Read the model definition and answer for the solid it produces. Units are mm, in the model's axes. Round coordinates to 2 decimals unless told otherwise and drop trailing zeros. Loops run counter-clockwise (first coordinate to the right, second up) from the corner with the lowest first, then second, coordinate; pieces in that order, holes last. Notation, with made-up numbers: (2, 20.25) - (23, 20.25) arc R37 ccw to (23, 56.25) - close; hole circle Ø3 at (-7, 54.5). An arc over 180 degrees is marked (long way). Use one line per item in the form item = value. Start each with the question number.
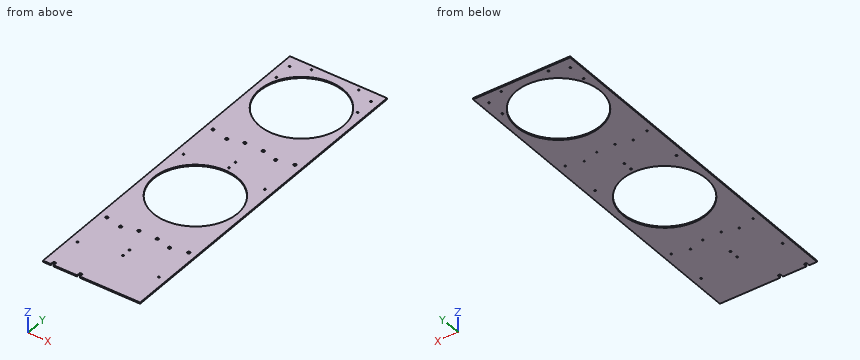
```python
from build123d import *

# Parameters (mm, degrees)
SKETCH1_W                                     = 469.9
SKETCH1_H                                     = 2413
SKETCH1_R                                     = 203.2
BOSS_EXTRUDE1_DEPTH                           = 6.35
CSK_FOR_1_4_FLAT_HEAD_SOCKET_CAP_SCR_2_COUNT  = 2
CSK_FOR_1_4_FLAT_HEAD_SOCKET_CAP_SCR_2_PITCH  = 76.2
CSK_FOR_1_4_FLAT_HEAD_SOCKET_CAP_SCR_3_COUNT  = 2
CSK_FOR_1_4_FLAT_HEAD_SOCKET_CAP_SCR_3_PITCH  = 89.142542345
CSK_FOR_1_4_FLAT_HEAD_SOCKET_CAP_SCR_4_COUNT  = 2
CSK_FOR_1_4_FLAT_HEAD_SOCKET_CAP_SCR_4_PITCH  = 163.936718394
CSK_FOR_1_4_FLAT_HEAD_SOCKET_CAP_SCR_5_COUNT  = 2
CSK_FOR_1_4_FLAT_HEAD_SOCKET_CAP_SCR_5_PITCH  = 711.2
CSK_FOR_1_4_FLAT_HEAD_SOCKET_CAP_SCR_6_COUNT  = 2
CSK_FOR_1_4_FLAT_HEAD_SOCKET_CAP_SCR_6_PITCH  = 695.384275934
CSK_FOR_1_4_FLAT_HEAD_SOCKET_CAP_SCR_7_COUNT  = 2
CSK_FOR_1_4_FLAT_HEAD_SOCKET_CAP_SCR_7_PITCH  = 716.764837904
CSK_FOR_1_4_FLAT_HEAD_SOCKET_CAP_SCR_8_COUNT  = 2
CSK_FOR_1_4_FLAT_HEAD_SOCKET_CAP_SCR_8_PITCH  = 710.371803251
CSK_FOR_1_4_FLAT_HEAD_SOCKET_CAP_SCR_9_COUNT  = 2
CSK_FOR_1_4_FLAT_HEAD_SOCKET_CAP_SCR_9_PITCH  = 1422.4
CSK_FOR_1_4_FLAT_HEAD_SOCKET_CAP_SCR_10_COUNT = 2
CSK_FOR_1_4_FLAT_HEAD_SOCKET_CAP_SCR_10_PITCH = 1404.60778242
CSK_FOR_1_4_FLAT_HEAD_SOCKET_CAP_SCR_11_COUNT = 2
CSK_FOR_1_4_FLAT_HEAD_SOCKET_CAP_SCR_11_PITCH = 1425.190567207
CSK_FOR_1_4_FLAT_HEAD_SOCKET_CAP_SCR_12_COUNT = 2
CSK_FOR_1_4_FLAT_HEAD_SOCKET_CAP_SCR_12_PITCH = 1412.087755797
CSK_FOR_1_4_FLAT_HEAD_SOCKET_CAP_SCR_13_COUNT = 2
CSK_FOR_1_4_FLAT_HEAD_SOCKET_CAP_SCR_13_PITCH = 153.55813077
CSK_FOR_1_4_FLAT_HEAD_SOCKET_CAP_SCR_14_COUNT = 2
CSK_FOR_1_4_FLAT_HEAD_SOCKET_CAP_SCR_14_PITCH = 242.697219812
CSK_FOR_1_4_FLAT_HEAD_SOCKET_CAP_SCR_15_COUNT = 2
CSK_FOR_1_4_FLAT_HEAD_SOCKET_CAP_SCR_15_PITCH = 749.86024568
CSK_FOR_1_4_FLAT_HEAD_SOCKET_CAP_SCR_16_COUNT = 2
CSK_FOR_1_4_FLAT_HEAD_SOCKET_CAP_SCR_16_PITCH = 1441.280581843
CSK_FOR_1_4_FLAT_HEAD_SOCKET_CAP_SCR_17_COUNT = 2
CSK_FOR_1_4_FLAT_HEAD_SOCKET_CAP_SCR_17_PITCH = 1428.974413563
CSK_FOR_1_4_FLAT_HEAD_SOCKET_CAP_SCR_18_COUNT = 2
CSK_FOR_1_4_FLAT_HEAD_SOCKET_CAP_SCR_18_PITCH = 725.925992834
F_5_16_0_3125_DIAMETER_HOLE1_D                = 7.9375
SKETCH6_W                                     = 469.9
SKETCH6_H                                     = 758.19
CUT_EXTRUDE1_DEPTH                            = 7.35
SKETCH8_W                                     = 13.208
SKETCH8_H                                     = 19.05
CUT_EXTRUDE2_DEPTH                            = 7.35
FILLET1_R                                     = 3.175


with BuildPart() as part:
    # Sketch1 → Boss-Extrude1 (new body)
    with BuildSketch(Plane.XY):
        with Locations((0, 1206.5)):
            Rectangle(SKETCH1_W, SKETCH1_H)
        with Locations((0, 695.96)):
            Circle(SKETCH1_R, mode=Mode.SUBTRACT)
        with Locations((0, 1407.16)):
            Circle(SKETCH1_R, mode=Mode.SUBTRACT)
        with Locations((0, 2118.36)):
            Circle(SKETCH1_R, mode=Mode.SUBTRACT)
    extrude(amount=BOSS_EXTRUDE1_DEPTH)

    # Sketch3 → CSK for 1/4 Flat Head Socket Cap Screw1 (revolve, cut)
    with BuildSketch(Plane(origin=(44.571271172, 378.545152647, 6.35), x_dir=(0, -1, 0), z_dir=(1, 0, 0))):
        Polygon((0, 0), (0, 6.35), (3.3782, 6.35), (3.3782, 3.871564875), (6.7437, 0), align=None)
    csk_for_1_4_flat_head_socket_cap_screw1 = revolve(axis=Axis((44.571271172, 378.545152647, 12.7), (0, 0, -1)), mode=Mode.SUBTRACT)

    # CSK for 1_4 Flat Head Socket Cap Scr 2: CSK for 1/4 Flat Head Socket Cap Screw1 ×2
    with Locations(*[Vector(0.965925826, -0.258819045, 0) * (i * CSK_FOR_1_4_FLAT_HEAD_SOCKET_CAP_SCR_2_PITCH) for i in range(1, CSK_FOR_1_4_FLAT_HEAD_SOCKET_CAP_SCR_2_COUNT)]):
        add(csk_for_1_4_flat_head_socket_cap_screw1, mode=Mode.SUBTRACT)

    # CSK for 1_4 Flat Head Socket Cap Scr 3: CSK for 1/4 Flat Head Socket Cap Screw1 ×2
    with Locations(*[(-i * CSK_FOR_1_4_FLAT_HEAD_SOCKET_CAP_SCR_3_PITCH, 0, 0) for i in range(1, CSK_FOR_1_4_FLAT_HEAD_SOCKET_CAP_SCR_3_COUNT)]):
        add(csk_for_1_4_flat_head_socket_cap_screw1, mode=Mode.SUBTRACT)

    # CSK for 1_4 Flat Head Socket Cap Scr 4: CSK for 1/4 Flat Head Socket Cap Screw1 ×2
    with Locations(*[Vector(-0.99273727, -0.120302586, 0) * (i * CSK_FOR_1_4_FLAT_HEAD_SOCKET_CAP_SCR_4_PITCH) for i in range(1, CSK_FOR_1_4_FLAT_HEAD_SOCKET_CAP_SCR_4_COUNT)]):
        add(csk_for_1_4_flat_head_socket_cap_screw1, mode=Mode.SUBTRACT)

    # CSK for 1_4 Flat Head Socket Cap Scr 5: CSK for 1/4 Flat Head Socket Cap Screw1 ×2
    with Locations(*[(0, i * CSK_FOR_1_4_FLAT_HEAD_SOCKET_CAP_SCR_5_PITCH, 0) for i in range(1, CSK_FOR_1_4_FLAT_HEAD_SOCKET_CAP_SCR_5_COUNT)]):
        add(csk_for_1_4_flat_head_socket_cap_screw1, mode=Mode.SUBTRACT)

    # CSK for 1_4 Flat Head Socket Cap Scr 6: CSK for 1/4 Flat Head Socket Cap Screw1 ×2
    with Locations(*[Vector(0.105845862, 0.994382549, 0) * (i * CSK_FOR_1_4_FLAT_HEAD_SOCKET_CAP_SCR_6_PITCH) for i in range(1, CSK_FOR_1_4_FLAT_HEAD_SOCKET_CAP_SCR_6_COUNT)]):
        add(csk_for_1_4_flat_head_socket_cap_screw1, mode=Mode.SUBTRACT)

    # CSK for 1_4 Flat Head Socket Cap Scr 7: CSK for 1/4 Flat Head Socket Cap Screw1 ×2
    with Locations(*[Vector(-0.124367907, 0.992236173, 0) * (i * CSK_FOR_1_4_FLAT_HEAD_SOCKET_CAP_SCR_7_PITCH) for i in range(1, CSK_FOR_1_4_FLAT_HEAD_SOCKET_CAP_SCR_7_COUNT)]):
        add(csk_for_1_4_flat_head_socket_cap_screw1, mode=Mode.SUBTRACT)

    # CSK for 1_4 Flat Head Socket Cap Scr 8: CSK for 1/4 Flat Head Socket Cap Screw1 ×2
    with Locations(*[Vector(-0.229099874, 0.973402922, 0) * (i * CSK_FOR_1_4_FLAT_HEAD_SOCKET_CAP_SCR_8_PITCH) for i in range(1, CSK_FOR_1_4_FLAT_HEAD_SOCKET_CAP_SCR_8_COUNT)]):
        add(csk_for_1_4_flat_head_socket_cap_screw1, mode=Mode.SUBTRACT)

    # CSK for 1_4 Flat Head Socket Cap Scr 9: CSK for 1/4 Flat Head Socket Cap Screw1 ×2
    with Locations(*[(0, i * CSK_FOR_1_4_FLAT_HEAD_SOCKET_CAP_SCR_9_PITCH, 0) for i in range(1, CSK_FOR_1_4_FLAT_HEAD_SOCKET_CAP_SCR_9_COUNT)]):
        add(csk_for_1_4_flat_head_socket_cap_screw1, mode=Mode.SUBTRACT)

    # CSK for 1_4 Flat Head Socket Cap Scr 10: CSK for 1/4 Flat Head Socket Cap Screw1 ×2
    with Locations(*[Vector(0.052401495, 0.998626098, 0) * (i * CSK_FOR_1_4_FLAT_HEAD_SOCKET_CAP_SCR_10_PITCH) for i in range(1, CSK_FOR_1_4_FLAT_HEAD_SOCKET_CAP_SCR_10_COUNT)]):
        add(csk_for_1_4_flat_head_socket_cap_screw1, mode=Mode.SUBTRACT)

    # CSK for 1_4 Flat Head Socket Cap Scr 11: CSK for 1/4 Flat Head Socket Cap Screw1 ×2
    with Locations(*[Vector(-0.062547805, 0.998041969, 0) * (i * CSK_FOR_1_4_FLAT_HEAD_SOCKET_CAP_SCR_11_PITCH) for i in range(1, CSK_FOR_1_4_FLAT_HEAD_SOCKET_CAP_SCR_11_COUNT)]):
        add(csk_for_1_4_flat_head_socket_cap_screw1, mode=Mode.SUBTRACT)

    # CSK for 1_4 Flat Head Socket Cap Scr 12: CSK for 1/4 Flat Head Socket Cap Screw1 ×2
    with Locations(*[Vector(-0.115252108, 0.993336273, 0) * (i * CSK_FOR_1_4_FLAT_HEAD_SOCKET_CAP_SCR_12_PITCH) for i in range(1, CSK_FOR_1_4_FLAT_HEAD_SOCKET_CAP_SCR_12_COUNT)]):
        add(csk_for_1_4_flat_head_socket_cap_screw1, mode=Mode.SUBTRACT)

    # CSK for 1_4 Flat Head Socket Cap Scr 13: CSK for 1/4 Flat Head Socket Cap Screw1 ×2
    with Locations(*[Vector(0.999938773, -0.011065747, 0) * (i * CSK_FOR_1_4_FLAT_HEAD_SOCKET_CAP_SCR_13_PITCH) for i in range(1, CSK_FOR_1_4_FLAT_HEAD_SOCKET_CAP_SCR_13_COUNT)]):
        add(csk_for_1_4_flat_head_socket_cap_screw1, mode=Mode.SUBTRACT)

    # CSK for 1_4 Flat Head Socket Cap Scr 14: CSK for 1/4 Flat Head Socket Cap Screw1 ×2
    with Locations(*[Vector(-0.999975489, -0.007001462, 0) * (i * CSK_FOR_1_4_FLAT_HEAD_SOCKET_CAP_SCR_14_PITCH) for i in range(1, CSK_FOR_1_4_FLAT_HEAD_SOCKET_CAP_SCR_14_COUNT)]):
        add(csk_for_1_4_flat_head_socket_cap_screw1, mode=Mode.SUBTRACT)

    # CSK for 1_4 Flat Head Socket Cap Scr 15: CSK for 1/4 Flat Head Socket Cap Screw1 ×2
    with Locations(*[Vector(-0.32364867, 0.946177329, 0) * (i * CSK_FOR_1_4_FLAT_HEAD_SOCKET_CAP_SCR_15_PITCH) for i in range(1, CSK_FOR_1_4_FLAT_HEAD_SOCKET_CAP_SCR_15_COUNT)]):
        add(csk_for_1_4_flat_head_socket_cap_screw1, mode=Mode.SUBTRACT)

    # CSK for 1_4 Flat Head Socket Cap Scr 16: CSK for 1/4 Flat Head Socket Cap Screw1 ×2
    with Locations(*[Vector(-0.168385861, 0.985721158, 0) * (i * CSK_FOR_1_4_FLAT_HEAD_SOCKET_CAP_SCR_16_PITCH) for i in range(1, CSK_FOR_1_4_FLAT_HEAD_SOCKET_CAP_SCR_16_COUNT)]):
        add(csk_for_1_4_flat_head_socket_cap_screw1, mode=Mode.SUBTRACT)

    # CSK for 1_4 Flat Head Socket Cap Scr 17: CSK for 1/4 Flat Head Socket Cap Screw1 ×2
    with Locations(*[Vector(0.107453799, 0.994210079, 0) * (i * CSK_FOR_1_4_FLAT_HEAD_SOCKET_CAP_SCR_17_PITCH) for i in range(1, CSK_FOR_1_4_FLAT_HEAD_SOCKET_CAP_SCR_17_COUNT)]):
        add(csk_for_1_4_flat_head_socket_cap_screw1, mode=Mode.SUBTRACT)

    # CSK for 1_4 Flat Head Socket Cap Scr 18: CSK for 1/4 Flat Head Socket Cap Screw1 ×2
    with Locations(*[Vector(0.211521189, 0.977373412, 0) * (i * CSK_FOR_1_4_FLAT_HEAD_SOCKET_CAP_SCR_18_PITCH) for i in range(1, CSK_FOR_1_4_FLAT_HEAD_SOCKET_CAP_SCR_18_COUNT)]):
        add(csk_for_1_4_flat_head_socket_cap_screw1, mode=Mode.SUBTRACT)

    # 5/16 (0.3125) Diameter Hole1 (through all)
    with Locations(Plane.XY.offset(6.35)):
        with Locations((0, 254.635), (0, 210.185), (-196.85, 177.8), (196.85, 177.8), (0, 965.835), (0, 921.385), (-196.85, 889), (196.85, 889), (-196.85, 1600.2), (196.85, 1600.2), (-114.3, 1632.585), (-114.3, 1677.035), (114.3, 1677.035), (114.3, 1632.585), (196.85, 1511.3), (-196.85, 1511.3)):
            Hole(F_5_16_0_3125_DIAMETER_HOLE1_D / 2)

    # Sketch6 → Cut-Extrude1 (cut, through all)
    with BuildSketch(Plane.XY.offset(6.35)):
        with Locations((0, 2033.905)):
            Rectangle(SKETCH6_W, SKETCH6_H)
    extrude(amount=-CUT_EXTRUDE1_DEPTH, mode=Mode.SUBTRACT)

    # Sketch8 → Cut-Extrude2 (cut, through all)
    with BuildSketch(Plane.XY.offset(6.35)):
        with Locations((-63.5, 9.525)):
            Rectangle(SKETCH8_W, SKETCH8_H)
        with Locations((-190.5, 9.525)):
            Rectangle(SKETCH8_W, SKETCH8_H)
    extrude(amount=-CUT_EXTRUDE2_DEPTH, mode=Mode.SUBTRACT)

    # Fillet1
    fillet1_edges = [part.edges().sort_by_distance(p)[0] for p in [
        (-70.104, 19.05, 3.175),
        (-56.896, 19.05, 3.175),
        (-197.104, 19.05, 3.175),
        (-183.896, 19.05, 3.175),
    ]]
    fillet(fillet1_edges, radius=FILLET1_R)


solid = part.part
```
1) Straight lines are drawn through the part: line 1 (Y direction, x = -157.5, z = 4); line 2 (X direction, y = 760, z = 3); line 3 (Y direction, x = -121.5, z = 4). For each, find the intervals that lie inside material, in ascending order. Write a range as from..to.
2) A cutting plane is placed at A-A on y = 695.96. Write down the section's boundary in (x, z).
3) Flat-ended cylindrical pins translate along their axes: pin 1 (12.5 mm diameter, centred on x = 0, y = 965.835, fed in from -Z); pin 2 (9 mm diameter, centred on x = 44.57, y = 1089.75, fed in from +Z). Find the tip coordinate at first contact, or state that the pin passes through.
4) A cutting plane is placed at C-C on y = 1359.5. Write down the section's boundary in (x, z), plus the area to 3 significant figures.
5) A cutting plane is placed at D-D on z = 3.75. Count the separate pieces of the cut face and the enclosed holes in it, plus the area to 3 significant figures.
6) A cutting plane is placed at B-B on x = 90. Write down the section's boundary in (y, z).
Checks:
q1.line_1 = 0..567.57, 824.35..1278.77, 1535.55..1654.81
q1.line_2 = -234.95..-192.84, 192.84..234.95
q1.line_3 = 0..355.5, 362.15..533.09, 858.83..1066.7, 1073.35..1244.29, 1570.03..1654.81
q2.outline = (-234.95, 0) - (-203.2, 0) - (-203.2, 6.35) - (-234.95, 6.35) - close; (203.2, 0) - (234.95, 0) - (234.95, 6.35) - (203.2, 6.35) - close
q3.pin_1 = 0
q3.pin_2 = 3.77
q4.outline = (-234.95, 0) - (-197.53, 0) - (-197.53, 6.35) - (-234.95, 6.35) - close; (197.53, 0) - (234.95, 0) - (234.95, 6.35) - (197.53, 6.35) - close
q4.area = 475 mm²
q5.separate_pieces = 1
q5.enclosed_holes = 28
q5.area = 516,000 mm²
q6.outline = (0, 0) - (513.78, 0) - (513.78, 6.35) - (0, 6.35) - close; (878.14, 0) - (1224.98, 0) - (1224.98, 6.35) - (878.14, 6.35) - close; (1589.34, 0) - (1654.81, 0) - (1654.81, 6.35) - (1589.34, 6.35) - close
